```python
from build123d import *

# Parameters (mm, degrees)
F1_DEPTH = 60
F2_R     = 12
F3_DEPTH = 60.001
F5_DEPTH = 40.001
F7_DEPTH = 73.386132
F8_W     = 22
F8_H     = 14
F9_DEPTH = 120.001


with BuildPart() as f1:
    # F0 (on Front) → F1 (new body)
    with BuildSketch(Plane.XZ):
        Polygon((-25, -8.385132), (-25, -25), (25, -25), (25, 25), (-25, 25), align=None)
        Polygon((-75, -25), (-25, -25), (-25, -8.385132), (-95, -8.385132), (-95, -48.385132), (-75, -48.385132), align=None)
    extrude(amount=F1_DEPTH)

    # F2 (on face) → F3 (cut, through all)
    with BuildSketch(Plane.XZ.offset(60)):
        Circle(F2_R)
    extrude(amount=-F3_DEPTH, mode=Mode.SUBTRACT)

    # F4 (on face) → F5 (cut, through all)
    with BuildSketch(Plane.XY.offset(-8.385132)):
        Polygon((-95, -44), (-65, -44), (-65, -16), (-125, -16), (-125, -44), align=None)
        with BuildLine():
            ThreePointArc((-15, -45), (-13.535534, -48.535534), (-10, -50))
            Line((-10, -50), (10, -50))
            ThreePointArc((10, -50), (13.535534, -48.535534), (15, -45))
            Line((15, -45), (15, -15))
            ThreePointArc((15, -15), (13.535534, -11.464466), (10, -10))
            Line((10, -10), (-10, -10))
            ThreePointArc((-10, -10), (-13.535534, -11.464466), (-15, -15))
            Line((-15, -15), (-15, -45))
        make_face()
    extrude(amount=-F5_DEPTH, mode=Mode.SUBTRACT)

    # F6 (on face) → F7 (cut, through all)
    with BuildSketch(Plane.XY.offset(25)):
        with BuildLine():
            ThreePointArc((-15, -45), (-13.535534, -48.535534), (-10, -50))
            Line((-10, -50), (10, -50))
            ThreePointArc((10, -50), (13.535534, -48.535534), (15, -45))
            Line((15, -45), (15, -15))
            ThreePointArc((15, -15), (13.535534, -11.464466), (10, -10))
            Line((10, -10), (-10, -10))
            ThreePointArc((-10, -10), (-13.535534, -11.464466), (-15, -15))
            Line((-15, -15), (-15, -45))
        make_face()
    extrude(amount=-F7_DEPTH, mode=Mode.SUBTRACT)

    # F8 (on face) → F9 (cut, through all)
    with BuildSketch(Plane.YZ.offset(25)):
        with Locations((-30, 8)):
            Rectangle(F8_W, F8_H)
    extrude(amount=-F9_DEPTH, mode=Mode.SUBTRACT)


solid = f1.part
```
Source: CAD feature listing. Evaluate the final solid. Frame: model axes, mm. A direction names the side the tool comes from. Round coordinates to 2 decimals unless told otherwise and drop trailing zeros. Loops run counter-clockwise (first coordinate to the right, second up) from the corner with the lowest first, then second, coordinate; pieces in that order, holes last.
(1) Section query B-B (y = -31). Output: boundary loops of the cut face in (x, z).
From the geometry:
outline: (-65, -25) - (-15, -25) - (-15, 1) - (-25, 1) - (-25, -8.39) - (-65, -8.39) - close; (-25, 15) - (-15, 15) - (-15, 25) - (-25, 25) - close; (15, -25) - (25, -25) - (25, 1) - (15, 1) - close; (15, 15) - (25, 15) - (25, 25) - (15, 25) - close
(2) Pull-direction query (Y, two-part tool) for faces 1 (the flat face through (-95, -52, -28)), 2 (the flat face through (20, -30, 1)), 3 (the flat face through (-36, -60, -11)); classes: +Y half, -Y half, draft (parallel to the pull), parting line (faces both ways), or undercut.
From the geometry:
face 1: draft
face 2: undercut
face 3: -Y half
(3) Section query D-D (x = -82.5). Output: boundary loops of the cut face in (y, z), and give its area (3 significant figures).
From the geometry:
outline: (-60, -48.39) - (-44, -48.39) - (-44, -8.39) - (-60, -8.39) - close; (-16, -48.39) - (0, -48.39) - (0, -8.39) - (-16, -8.39) - close
area: 1,280 mm2
(4) Section query A-A (z = -27.5). Output: boundary loops of the cut face in (x, y), and give its area (3 significant figures).
From the geometry:
outline: (-95, -60) - (-75, -60) - (-75, -44) - (-95, -44) - close; (-95, -16) - (-75, -16) - (-75, 0) - (-95, 0) - close
area: 640 mm2
(5) Material intervals for probe 1 along X at (y, z) = (-3.25, 0); probe 2 along X at (y, z) = (-16.5, 1), sorted ascending.
From the geometry:
probe 1: x = -25 to -12, 12 to 25
probe 2: x = -25 to -15, 15 to 25
(6) Section query C-C (x = 0). Output: boundary loops of the cut face in (y, z).
From the geometry:
outline: (-60, -25) - (-50, -25) - (-50, -12) - (-60, -12) - close; (-60, 12) - (-50, 12) - (-50, 25) - (-60, 25) - close; (-10, -25) - (0, -25) - (0, -12) - (-10, -12) - close; (-10, 12) - (0, 12) - (0, 25) - (-10, 25) - close
(7) Contact query for flat-ended pins moving along their axis: pin 1 Ø1 at (x, z) = (-70.5, -18) entering from +Y; pin 2 Ø8 at (y, z) = (-11, -40.5) entering from +X; pin 3 Ø9 at (y, z) = (-28, -7) entering from -X; pin 4 Ø2 at (x, y) = (-23, -22) entering from -Z. Output: stop coordinate, or through.
From the geometry:
pin 1: stops at y = 0
pin 2: stops at x = -75
pin 3: stops at x = -65
pin 4: stops at z = -25
(8) Access query for faces 4 (the flat face through (-65, -30, -17)), 5 (the flat face through (20, -19, 8)), 6 (the cylindrical face through (-11.99, -5.28, 0.53)), 7 (the flat face through (15, -30, 0)). Directions: +Z, -Z, +X, -X, +Y, -Y. A direction counts if a zero-diameter tool reaches every point of the face in a straight line with its end or side. Return the directions, or none.
From the geometry:
face 4: +Z, -Z, -X
face 5: +X, -X
face 6: +Y, -Y
face 7: +Z, -Z
